```python
from build123d import *

# Parameters (mm, degrees)
F0_W     = 115
F0_H     = 85
F0_W_2   = 12.42488157
F0_H_2   = 2.8554350138
F1_DEPTH = 3
F2_R     = 2.6556349186
F3_D     = 3.3
F3_DEPTH = 13.5
F3_TIP   = 0.9914200214


with BuildPart() as f1:
    # F0 (on Top) → F1 (new body)
    with BuildSketch(Plane.XY):
        Rectangle(F0_W, F0_H)
        with Locations((0.012440607, -39.7679619491)):
            Rectangle(F0_W_2, F0_H_2, mode=Mode.SUBTRACT)
        with Locations((0.1124413684, 39.7277288139)):
            Rectangle(F0_W_2, F0_H_2, mode=Mode.SUBTRACT)
    extrude(amount=-F1_DEPTH)

    # F2
    f2_edges = [f1.edges().sort_by_distance(p)[0] for p in [
        (57.5, -42.5, -1.5),
        (57.5, 42.5, -1.5),
        (-57.5, -42.5, -1.5),
        (-57.5, 42.5, -1.5),
    ]]
    fillet(f2_edges, radius=F2_R)

    # F3
    with Locations(Plane.XY):
        with Locations((-53.4860491753, -38.9412779514), (-53.4860491753, 39.0123836696), (53.5768903792, -38.9412779514), (53.5768903792, 39.0123836696)):
            Hole(F3_D / 2, depth=F3_DEPTH)
            with Locations((0, 0, -(F3_DEPTH + F3_TIP / 2))):  # 118° drill point
                Cone(0, F3_D / 2, F3_TIP, mode=Mode.SUBTRACT)


solid = f1.part
```
Read the model definition and answer for the solid it produces. Units are mm, in the model's axes. A direction names the side the tool comes from. Give positions to 0.01 mm unless a question says otherwise; leave off trailing zeros.
(1) Given pin 1 (2.5 mm diameter, centred on x = 53.58, y = 39.01, fed in from -Z), flat-ended and moving along its own axis, determine where the tip first touches the part or whether it passes through.
(2) For faces 5 (the flat face through (6.225, -40, -1)), 6 (the cylindrical face through (56.701, -41.743, -1.521)), determine the directions among +Z, -Z, +X, -X, +Y, -Y from which every point of the face is accessible in a straight line to the end or side of a thin tool.
(3) For a pull along Y with two mould halves and no side action, classify faces 1 (the cylindrical face through (-55.01, 38.38, -1.52)), 2 (the flat face through (-1, -42.5, -1)), 3 (the flat face through (-57.5, -1, -1)), 4 (the flat face through (0, 41.155, -1)) as released by +Y, released by -Y, zero draft, split by the parting line, or undercut.
(4) Straight lines are drawn through the part: L1, parallel to Y at x = -1, z = -0.8; L2, parallel to X at y = -39, z = -2.1 (3 decimals). For each, find the intervals that lie inside material, in ascending order.
Result sheet:
1. pin 1: passes through
2. face 5: +Z, -Z
2. face 6: +Z, -Z, +X, -Y
3. face 1: undercut
3. face 2: released by -Y
3. face 3: zero draft
3. face 4: undercut
4. L1: y = -42.5 to -41.2, -38.34 to 38.3, 41.16 to 42.5
4. L2: x = -57.5 to -55.135, -51.837 to -6.2, 6.225 to 51.928, 55.226 to 57.5
